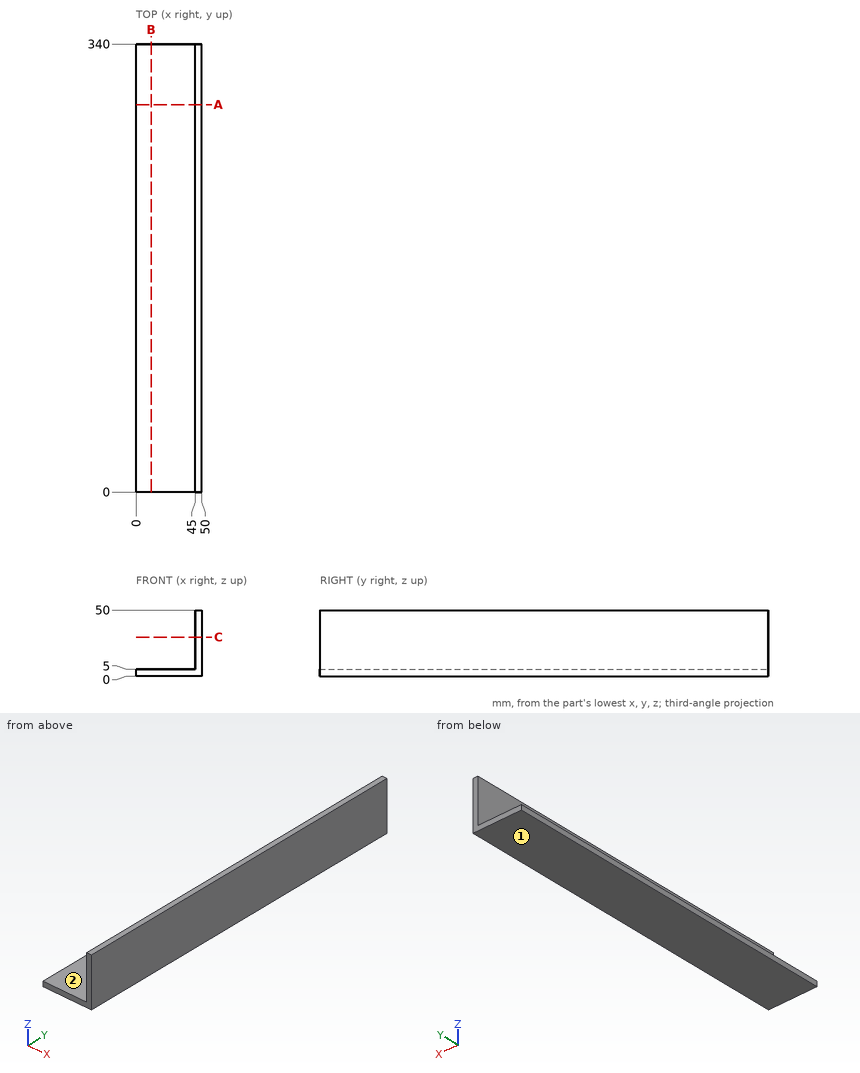
Here's the drawing with two shaded views (mm, measured from the low corner). I have some questions. A direction names the side the tool comes from. Give positions to 0.01 mm unless a question says otherwise; leave off trailing zeros. Order: outer loops, then holes, each group sorted by start corner. A loop starts at its lowest first (then second) coordinate and runs counter-clockwise, first axis right, second up. Notation, with made-up numbers: (62.25, 70) -> (96.25, 70) arc R21 cw to (96.25, 96) -> close; hole circle Ø9 at (-12, -19.5). An arc over 180 degrees is marked (long way). Use a Markdown table: item, result. Add a question column.
Item 1: Imagine slicing it at A-A on y = 294. Please give me the cut outline in (x, z).
Item 2: Imagine slicing it at C-C on z = 29.5. Please give me the cut outline in (x, y), plus the area to 3 significant figures.
Item 3: For the marked faces 1 and 2, which set-ups out of +Z, -Z, +X, -X, +Y, -Y let a thin tool reach every point of the face, with its end or its side?
Item 4: I need wall thicknesses on line 1 (Z direction, x = 26, y = 324); line 2 (X direction, y = 200.5, z = 14). Which ranges of each line are inside material? Lowest first, please.
Item 5: Imagine slicing it at B-B on x = 11.5. Please give me the cut outline in (y, z).
Item 6: Will these pins go through, and if not, where does the flat tip stop? pin 1 (1.5 mm diameter, centred on y = 111, z = 37.5, fed in from -X); pin 2 (13.5 mm diameter, centred on x = 11.5, y = 153.5, fed in from +Z); pin 3 (8 mm diameter, centred on x = 31.5, y = 118.5, fed in from -Z); pin 4 (4 mm diameter, centred on x = 42.5, z = 34, fed in from -Y).
Data:
| question | item | result |
|---|---|---|
| 1 | outline | (0, 0) -> (50, 0) -> (50, 50) -> (45, 50) -> (45, 5) -> (0, 5) -> close |
| 2 | outline | (45, 0) -> (50, 0) -> (50, 340) -> (45, 340) -> close |
| 2 | area | 1,700 mm² |
| 3 | face 1 | -Z, +X, -X, +Y, -Y |
| 3 | face 2 | +Z, -X, +Y, -Y |
| 4 | line 1 | z = 0 to 5 |
| 4 | line 2 | x = 45 to 50 |
| 5 | outline | (0, 0) -> (340, 0) -> (340, 5) -> (0, 5) -> close |
| 6 | pin 1 | stops at x = 45 |
| 6 | pin 2 | stops at z = 5 |
| 6 | pin 3 | stops at z = 0 |
| 6 | pin 4 | passes through |
